Design review of the part built by this model. Coordinates are the model's own, in mm. Coordinates: 2 decimals unless noted, no trailing zeros. Order: outer loops, then holes, each group sorted by start corner. A loop starts at its lowest first (then second) coordinate and runs counter-clockwise, first axis right, second up. Notation, with made-up numbers: M 13,56.25 L 31,56.25 A33 ccw 31,85.25 Z; hole C -36,85 d9. An arc over 180 degrees is marked long. Answer as a JSON object with one key per item and string values.
from build123d import *

# Parameters (mm, degrees)
F0_W     = 381
F0_H     = 381
F0_R     = 82.55
F1_DEPTH = 50.8


with BuildPart() as f1:
    # F0 (on Right) → F1 (new body, symmetric)
    with BuildSketch(Plane.YZ):
        with Locations((190.5, -190.5)):
            Rectangle(F0_W, F0_H)
        with Locations((190.5, -190.5)):
            Circle(F0_R, mode=Mode.SUBTRACT)
    extrude(amount=F1_DEPTH, both=True)


solid = f1.part
1) Add section B-B (z = -190.5). State the section outline as (x, y) points.
Taken from the geometry:
{"outline": "M -50.8,0 L 50.8,0 L 50.8,107.95 L -50.8,107.95 Z; M -50.8,273.05 L 50.8,273.05 L 50.8,381 L -50.8,381 Z"}
2) Add section C-C (x = -22.5). State the section outline as (y, z) points.
Taken from the geometry:
{"outline": "M 0,-381 L 381,-381 L 381,0 L 0,0 Z; hole C 190.5,-190.5 d165.1"}
3) To check wall thickness, follow L1, parallel to Z at x = -18, y = 190.5; L2, parallel to Y at x = 5, z = -190; L3, parallel to Y at x = -11.5, z = -232.5. State the ranges of each line that lie inside material, in increasing order.
Taken from the geometry:
{"L1": "z = -381 to -273.05, -107.95 to 0", "L2": "y = 0 to 107.95, 273.05 to 381", "L3": "y = 0 to 119.43, 261.57 to 381"}
4) Add section A-A (y = 190.5). State the section outline as (x, z) points.
Taken from the geometry:
{"outline": "M -50.8,-381 L 50.8,-381 L 50.8,-273.05 L -50.8,-273.05 Z; M -50.8,-107.95 L 50.8,-107.95 L 50.8,0 L -50.8,0 Z"}
5) Mouldability with a two-part tool opening along Y and no side actions: class faces 1 (the cylindrical face through (-0.711, 266.755, -222.117)), 2 (the flat face through (1, 188, -381)), 3 (the flat face through (1, 381, -193)), 4 (the flat face through (1, 0, -193)) as released by +Y, released by -Y, zero draft, split by the parting line, or undercut.
Taken from the geometry:
{"face 1": "undercut", "face 2": "zero draft", "face 3": "released by +Y", "face 4": "released by -Y"}
